from build123d import *

# Parameters (mm, degrees)
SKETCH3_W           = 200
SKETCH3_H           = 150
BOSS_EXTRUDE1_DEPTH = 100
BOSS_EXTRUDE1_TAPER = -1
FILLET1_R           = 5
SHELL1_T            = -3
SKETCH10_W          = 20
SKETCH10_H          = 25.4
SKETCH10_W_2        = 50
SKETCH10_H_2        = 20
CUT_EXTRUDE6_DEPTH  = 59.614
CUT_EXTRUDE6_TAPER  = -1
SKETCH12_W          = 63.5
SKETCH12_H          = 38.1
CUT_EXTRUDE7_DEPTH  = 100
CUT_EXTRUDE7_TAPER  = -1


with BuildPart() as part:
    # Sketch3 → Boss-Extrude1 (new body)
    with BuildSketch(Plane.XY):
        with Locations((-28.926930074, 63.110328622)):
            Rectangle(SKETCH3_W, SKETCH3_H)
    extrude(amount=BOSS_EXTRUDE1_DEPTH, taper=BOSS_EXTRUDE1_TAPER)

    # Fillet1
    fillet1_edges = [part.edges().sort_by_distance(p)[0] for p in [
        (71.945823172, -12.762424624, 50),
        (-129.799683321, -12.762424624, 50),
        (-129.799683321, 138.983081869, 50),
        (71.945823172, 138.983081869, 50),
    ]]
    fillet(fillet1_edges, radius=FILLET1_R)

    # Shell1
    shell1_openings = [part.faces().sort_by_distance(p)[0] for p in [
        (-28.926930074, 63.110328622, 100),
    ]]
    offset(amount=SHELL1_T, openings=shell1_openings, kind=Kind.INTERSECTION)

    # Sketch10 → Cut-Extrude6 (cut)
    with BuildSketch(Plane(origin=(0, 0, 0), x_dir=(-1, 0, 0), z_dir=(0, 0, -1))):
        with Locations((-41.331432063, 119.367467356)):
            Rectangle(SKETCH10_W, SKETCH10_H)
        with Locations((-38.825178327, 7.672208688)):
            Rectangle(SKETCH10_W_2, SKETCH10_H_2)
    extrude(amount=-CUT_EXTRUDE6_DEPTH, taper=CUT_EXTRUDE6_TAPER, mode=Mode.SUBTRACT)

    # Sketch12 → Cut-Extrude7 (cut)
    with BuildSketch(Plane(origin=(0, 0, 0), x_dir=(-1, 0, 0), z_dir=(0, 0, -1))):
        with Locations((90.091836521, 26.275420471)):
            Rectangle(SKETCH12_W, SKETCH12_H)
    extrude(amount=-CUT_EXTRUDE7_DEPTH, taper=CUT_EXTRUDE7_TAPER, mode=Mode.SUBTRACT)


solid = part.part
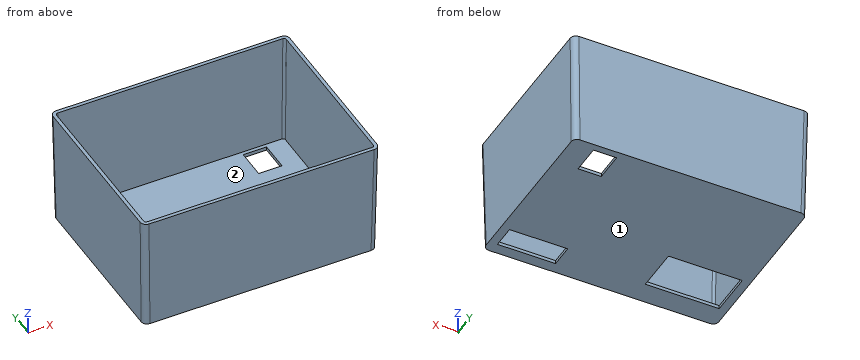
Model file for the job. Use its own axes, mm. Face numbers are marked on the shaded views. Coordinates: 2 decimals unless noted, no trailing zeros. Write each question's results on one line, items separated by ' | '. Start each with the question number.
1) Probe line 1 along Z through (x, y) = (-7.5, 69); line 2 along X through (y, z) = (-4, 16.5); line 3 along Y through (x, z) = (58.5, 76). List the from-to ranges inside material, lowest first. Write a range as from..to.
2) Mould opens along X. For the marked faces 1 and 2 say: pulls with the +X half, pulls with the -X half, needs draft (parallel to the pull), parting line crosses it, or undercut.
3) Flat gauge pins, fed straight in: P1, Ø10, axis at y = 35.5, z = 26, coming from the -X side; P2, Ø10, axis at x = -18, z = 44.5, coming from the -Y side; P3, Ø12, axis at y = 52, z = 13, coming from the -X side. Where does each tip first touch, or does it go through?
4) Cut at A-A (x = 41.5). Count the separate pieces of the cut face and the enclosed holes in it, then the cut area to 3 significant figures.
Returned:
1) line 1: 0..3 | line 2: -129.21..-126.21, 68.36..71.36 | line 3: -13.22..-10.22, 136.44..139.44
2) face 1: needs draft | face 2: undercut
3) P1: x = -129.47 | P2: y = -12.75 | P3: x = -129.26
4) separate pieces: 3 | enclosed holes: 0 | area: 896 mm^2
